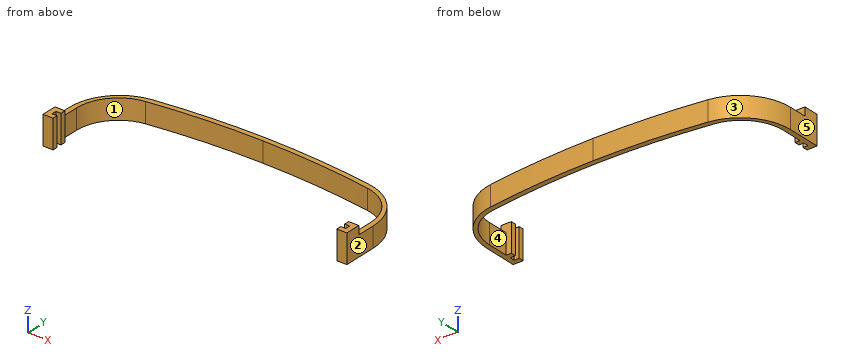
```python
from build123d import *

# Parameters (mm, degrees)
BOSS_EXTRUDE1_DEPTH = 12
BOSS_EXTRUDE2_DEPTH = 5
FILLET1_R           = 25
FILLET2_R           = 30


with BuildPart() as part:
    # Sketch1 → Boss-Extrude1 (new body)
    with BuildSketch(Plane.XY):
        with BuildLine():
            Line((84.5, 0), (87.5, 0))
            Line((87.5, 0), (87.5, 3))
            Line((87.5, 3), (84.5, 3))
            Line((84.5, 3), (84.5, 6))
            Line((84.5, 6), (87.5, 6))
            Line((87.5, 6), (87.5, 39.535975243))
            ThreePointArc((87.5, 39.535975243), (43.954208317, 45.879066954), (0, 48))
            Line((0, 48), (0, 51))
            ThreePointArc((0, 51), (45.473206397, 48.744464323), (90.5, 42))
            Line((90.5, 42), (90.5, -3))
            Line((90.5, -3), (84.5, -3))
            Line((84.5, -3), (84.5, 0))
        make_face()
    boss_extrude1 = extrude(amount=BOSS_EXTRUDE1_DEPTH)

    # Sketch2 → Boss-Extrude2 (add)
    with BuildSketch(Plane.XY.offset(12)):
        Polygon((90.5, -3), (84.5, -3), (84.5, 0), (87.5, 0), (87.5, 3), (84.5, 3), (84.5, 6), (90.5, 6), align=None)
    boss_extrude2 = extrude(amount=BOSS_EXTRUDE2_DEPTH)

    # Mirror1: Boss-Extrude1, Boss-Extrude2 across plane
    add(boss_extrude1.mirror(Plane(origin=(0, 0, 0), x_dir=(0, 0, 1), z_dir=(1, 0, 0))))
    add(boss_extrude2.mirror(Plane(origin=(0, 0, 0), x_dir=(0, 0, 1), z_dir=(1, 0, 0))))

    # Fillet1
    fillet1_edges = [part.edges().sort_by_distance(p)[0] for p in [
        (87.5, 39.535975243, 6),
        (-87.5, 39.535975243, 6),
    ]]
    fillet(fillet1_edges, radius=FILLET1_R)

    # Fillet2
    fillet2_edges = [part.edges().sort_by_distance(p)[0] for p in [
        (90.5, 42, 6),
        (-90.5, 42, 6),
    ]]
    fillet(fillet2_edges, radius=FILLET2_R)


solid = part.part
```
The listing builds one solid part. Answer for the finished solid, in the listing's coordinates (mm). Face numbers are marked on the shaded views. A direction names the side the tool comes from. Coordinates: 2 decimals unless noted, no trailing zeros. Write each loop counter-clockwise with the first axis right and the second up, starting at its lowest first coordinate (ties: lowest second). Pieces come first, ordered by that corner, then holes. Notation, with made-up numbers: (60, 7) - (96, 7) arc R27 cw to (96, 27) - close; hole circle Ø5 at (-8.5, -40). An arc over 180 degrees is marked (long way). Return JSON: item names as keys, results as strings. Group by question number.
1. Which of the six approach directions +Z, -Z, +X, -X, +Y, -Y give full straight-line access (tool end or side, diameter ignored) to the marked faces 4 and 5?
2. Straight lines are drawn through the part: L1, parallel to X at y = 4, z = 8.5; L2, parallel to X at y = 17, z = 5.25; L3, parallel to Z at x = 75.5, y = 42. For each, find the intervals that lie inside material, in ascending order.
3. A cutting plane is placed at B-B, the plane y = 8. Determine the outline of the cut face in (x, z).
4. Given pin 1 (2.5 mm diameter, centred on x = 85.5, z = 5.5, fed in from +Y); pin 2 (6 mm diameter, centred on y = 36, z = 8.5, fed in from +X); pin 3 (8 mm diameter, centred on y = 22, z = 12.5, fed in from -X); pin 4 (2 mm diameter, centred on x = 56.5, z = 14.5, fed in from +Y), each flat-ended and moving along its own axis, determine where each tip first touches the part or whether it passes through.
5. Determine the mould class of the marked faces 1, 2 and 3 for opening direction X: released by +X, released by -X, zero draft, split by the parting line, or undercut.
6. A cutting plane is placed at D-D, the plane x = -76. Determine the outline of the cut face in (y, z), plus the area to 3 significant figures.
7. A cutting plane is placed at C-C, the plane y = 25.5. Determine the outline of the cut face in (x, z).
8. A cutting plane is placed at A-A, the plane z = 14.5. Determine the outline of the cut face in (x, y), plus the area to 3 significant figures.
Ans:
{
 "1": {"face 4": "+Z, -Z", "face 5": "+Z, -Z, -X, +Y, -Y"},
 "2": {"L1": "-90.5 to -84.5, 84.5 to 90.5", "L2": "-90.5 to -87.5, 87.5 to 90.5", "L3": "0 to 12"},
 "3": {"outline": "(-90.5, 0) - (-87.5, 0) - (-87.5, 12) - (-90.5, 12) - close; (87.5, 0) - (90.5, 0) - (90.5, 12) - (87.5, 12) - close"},
 "4": {"pin 1": "y = 35.05", "pin 2": "x = 85.7", "pin 3": "x = -90.47", "pin 4": "through"},
 "5": {"face 1": "undercut", "face 2": "released by +X", "face 3": "released by -X"},
 "6": {"outline": "(39.49, 0) - (42.4, 0) - (42.4, 12) - (39.49, 12) - close", "area": "34.9 mm²"},
 "7": {"outline": "(-89.19, 0) - (-86.49, 0) - (-86.49, 12) - (-89.19, 12) - close; (86.49, 0) - (89.19, 0) - (89.19, 12) - (86.49, 12) - close"},
 "8": {"outline": "(-90.5, -3) - (-84.5, -3) - (-84.5, 0) - (-87.5, 0) - (-87.5, 3) - (-84.5, 3) - (-84.5, 6) - (-90.5, 6) - close; (84.5, -3) - (90.5, -3) - (90.5, 6) - (84.5, 6) - (84.5, 3) - (87.5, 3) - (87.5, 0) - (84.5, 0) - close", "area": "90.0 mm²"}
}
